```python
from build123d import *

# Parameters (mm, degrees)
F1_DEPTH = 609.6


with BuildPart() as f1:
    # F0 (on Right) → F1 (new body)
    with BuildSketch(Plane.YZ):
        with BuildLine():
            Line((-59.69, 12.737884), (-53.34, 12.737884))
            ThreePointArc((-53.34, 12.737884), (-56.515, 14.642884), (-59.69, 12.737884))
        make_face()
        with BuildLine():
            ThreePointArc((-118.11, 12.737884), (-121.285, 14.642884), (-124.46, 12.737884))
            Line((-124.46, 12.737884), (-118.11, 12.737884))
        make_face()
        with BuildLine():
            Line((-252.4125, 9.562884), (-9.525, 9.562884))
            ThreePointArc((-9.525, 9.562884), (-2.789808, 6.773076), (0, 0.037884))
            Line((0, 0.037884), (0, -11.720433))
            ThreePointArc((0, -11.720433), (-8.067335, -19.327291), (-15.187478, -10.827306))
            ThreePointArc((-15.187478, -10.827306), (-17.598242, -6.218379), (-22.768182, -6.789089))
            ThreePointArc((-22.768182, -6.789089), (-22.948389, -9.016326), (-20.72294, -9.217406))
            ThreePointArc((-20.72294, -9.217406), (-19.12196, -9.047525), (-18.340594, -10.45517))
            ThreePointArc((-18.340594, -10.45517), (-8.253725, -22.496816), (3.175, -11.720433))
            Line((3.175, -11.720433), (3.175, 0.037884))
            ThreePointArc((3.175, 0.037884), (-0.544744, 9.01814), (-9.525, 12.737884))
            Line((-9.525, 12.737884), (-20.32, 12.737884))
            Line((-20.32, 12.737884), (-21.082, 12.737884))
            Line((-21.082, 12.737884), (-21.844, 12.737884))
            Line((-21.844, 12.737884), (-22.606, 12.737884))
            Line((-22.606, 12.737884), (-23.368, 12.737884))
            Line((-23.368, 12.737884), (-24.13, 12.737884))
            Line((-24.13, 12.737884), (-24.892, 12.737884))
            Line((-24.892, 12.737884), (-25.654, 12.737884))
            Line((-25.654, 12.737884), (-26.416, 12.737884))
            Line((-26.416, 12.737884), (-27.178, 12.737884))
            Line((-27.178, 12.737884), (-27.94, 12.737884))
            Line((-27.94, 12.737884), (-53.34, 12.737884))
            Line((-53.34, 12.737884), (-59.69, 12.737884))
            Line((-59.69, 12.737884), (-85.09, 12.737884))
            Line((-85.09, 12.737884), (-85.852, 12.737884))
            Line((-85.852, 12.737884), (-86.614, 12.737884))
            Line((-86.614, 12.737884), (-87.376, 12.737884))
            Line((-87.376, 12.737884), (-88.138, 12.737884))
            Line((-88.138, 12.737884), (-88.9, 12.737884))
            Line((-88.9, 12.737884), (-89.662, 12.737884))
            Line((-89.662, 12.737884), (-90.424, 12.737884))
            Line((-90.424, 12.737884), (-91.186, 12.737884))
            Line((-91.186, 12.737884), (-91.948, 12.737884))
            Line((-91.948, 12.737884), (-92.71, 12.737884))
            Line((-92.71, 12.737884), (-118.11, 12.737884))
            Line((-118.11, 12.737884), (-124.46, 12.737884))
            Line((-124.46, 12.737884), (-149.86, 12.737884))
            Line((-149.86, 12.737884), (-150.622, 12.737884))
            Line((-150.622, 12.737884), (-151.384, 12.737884))
            Line((-151.384, 12.737884), (-152.146, 12.737884))
            Line((-152.146, 12.737884), (-152.908, 12.737884))
            Line((-152.908, 12.737884), (-153.67, 12.737884))
            Line((-153.67, 12.737884), (-154.432, 12.737884))
            Line((-154.432, 12.737884), (-155.194, 12.737884))
            Line((-155.194, 12.737884), (-155.956, 12.737884))
            Line((-155.956, 12.737884), (-156.718, 12.737884))
            Line((-156.718, 12.737884), (-157.48, 12.737884))
            Line((-157.48, 12.737884), (-182.88, 12.737884))
            Line((-182.88, 12.737884), (-189.23, 12.737884))
            Line((-189.23, 12.737884), (-214.63, 12.737884))
            Line((-214.63, 12.737884), (-215.392, 12.737884))
            Line((-215.392, 12.737884), (-216.154, 12.737884))
            Line((-216.154, 12.737884), (-216.916, 12.737884))
            Line((-216.916, 12.737884), (-217.678, 12.737884))
            Line((-217.678, 12.737884), (-218.44, 12.737884))
            Line((-218.44, 12.737884), (-219.202, 12.737884))
            Line((-219.202, 12.737884), (-219.964, 12.737884))
            Line((-219.964, 12.737884), (-220.726, 12.737884))
            Line((-220.726, 12.737884), (-221.488, 12.737884))
            Line((-221.488, 12.737884), (-222.25, 12.737884))
            Line((-222.25, 12.737884), (-247.65, 12.737884))
            Line((-247.65, 12.737884), (-254, 12.737884))
            Line((-254, 12.737884), (-254, 11.150384))
            ThreePointArc((-254, 11.150384), (-253.535032, 10.027852), (-252.4125, 9.562884))
        make_face()
        with BuildLine():
            ThreePointArc((-247.65, 12.737884), (-250.825, 14.642884), (-254, 12.737884))
            Line((-254, 12.737884), (-247.65, 12.737884))
        make_face()
        with BuildLine():
            ThreePointArc((-182.88, 12.737884), (-186.055, 14.642884), (-189.23, 12.737884))
            Line((-189.23, 12.737884), (-182.88, 12.737884))
        make_face()
        Polygon((-85.852, 12.737884), (-85.09, 12.737884), (-85.852, 13.753884), align=None)
        Polygon((-21.082, 12.737884), (-20.32, 12.737884), (-21.082, 13.753884), align=None)
        Polygon((-222.25, 13.753884), (-222.25, 12.737884), (-221.488, 12.737884), align=None)
        Polygon((-21.844, 12.737884), (-21.082, 12.737884), (-21.844, 13.753884), align=None)
        Polygon((-150.622, 13.753884), (-150.622, 12.737884), (-149.86, 12.737884), align=None)
        Polygon((-151.384, 13.753884), (-151.384, 12.737884), (-150.622, 12.737884), align=None)
        Polygon((-221.488, 13.753884), (-221.488, 12.737884), (-220.726, 12.737884), align=None)
        Polygon((-86.614, 12.737884), (-85.852, 12.737884), (-86.614, 13.753884), align=None)
        Polygon((-26.416, 12.737884), (-25.654, 12.737884), (-26.416, 13.753884), align=None)
        Polygon((-27.178, 12.737884), (-26.416, 12.737884), (-27.178, 13.753884), align=None)
        Polygon((-152.908, 13.753884), (-152.908, 12.737884), (-152.146, 12.737884), align=None)
        Polygon((-157.48, 13.753884), (-157.48, 12.737884), (-156.718, 12.737884), align=None)
        Polygon((-215.392, 13.753884), (-215.392, 12.737884), (-214.63, 12.737884), align=None)
        Polygon((-92.71, 13.753884), (-92.71, 12.737884), (-91.948, 12.737884), align=None)
        Polygon((-89.662, 12.737884), (-88.9, 12.737884), (-89.662, 13.753884), align=None)
        Polygon((-155.194, 13.753884), (-155.194, 12.737884), (-154.432, 12.737884), align=None)
        Polygon((-153.67, 13.753884), (-153.67, 12.737884), (-152.908, 12.737884), align=None)
        Polygon((-91.948, 12.737884), (-91.186, 12.737884), (-91.948, 13.753884), align=None)
        Polygon((-87.376, 12.737884), (-86.614, 12.737884), (-87.376, 13.753884), align=None)
        Polygon((-24.13, 12.737884), (-23.368, 12.737884), (-24.13, 13.753884), align=None)
        Polygon((-27.94, 12.737884), (-27.178, 12.737884), (-27.94, 13.753884), align=None)
        Polygon((-90.424, 12.737884), (-89.662, 12.737884), (-90.424, 13.753884), align=None)
        Polygon((-23.368, 12.737884), (-22.606, 12.737884), (-23.368, 13.753884), align=None)
        Polygon((-218.44, 13.753884), (-218.44, 12.737884), (-217.678, 12.737884), align=None)
        Polygon((-219.202, 13.753884), (-219.202, 12.737884), (-218.44, 12.737884), align=None)
        Polygon((-216.154, 13.753884), (-216.154, 12.737884), (-215.392, 12.737884), align=None)
        Polygon((-155.956, 13.753884), (-155.956, 12.737884), (-155.194, 12.737884), align=None)
        Polygon((-219.964, 13.753884), (-219.964, 12.737884), (-219.202, 12.737884), align=None)
        Polygon((-88.138, 12.737884), (-87.376, 12.737884), (-88.138, 13.753884), align=None)
        Polygon((-88.9, 12.737884), (-88.138, 12.737884), (-88.9, 13.753884), align=None)
        Polygon((-24.892, 12.737884), (-24.13, 12.737884), (-24.892, 13.753884), align=None)
        Polygon((-152.146, 13.753884), (-152.146, 12.737884), (-151.384, 12.737884), align=None)
        Polygon((-220.726, 13.753884), (-220.726, 12.737884), (-219.964, 12.737884), align=None)
        Polygon((-216.916, 13.753884), (-216.916, 12.737884), (-216.154, 12.737884), align=None)
        Polygon((-156.718, 13.753884), (-156.718, 12.737884), (-155.956, 12.737884), align=None)
        Polygon((-154.432, 13.753884), (-154.432, 12.737884), (-153.67, 12.737884), align=None)
        Polygon((-217.678, 13.753884), (-217.678, 12.737884), (-216.916, 12.737884), align=None)
        Polygon((-25.654, 12.737884), (-24.892, 12.737884), (-25.654, 13.753884), align=None)
        Polygon((-22.606, 12.737884), (-21.844, 12.737884), (-22.606, 13.753884), align=None)
        Polygon((-91.186, 12.737884), (-90.424, 12.737884), (-91.186, 13.753884), align=None)
    extrude(amount=F1_DEPTH)


solid = f1.part
```
Geometry check sheet. Reference: the model listing, model coordinates, mm. A direction names the side the tool comes from. Coordinates: 2 decimals unless noted, no trailing zeros. Write each loop counter-clockwise with the first axis right and the second up, starting at its lowest first coordinate (ties: lowest second). Pieces come first, ordered by that corner, then holes. Notation, with made-up numbers: M -27,82 L -19,82 A15 cw -19,90 Z; hole C 32,74.25 d7. An arc over 180 degrees is marked long. One line per item, written item: value. Start each with the question number.
(1) Tool access check on faces 1 (the face through (301, -40, 12.738)), 2 (the face through (609.6, -116, 10)), 3 (the face through (300.533, -7.894, -19.336)). Record the directions out of +Z, -Z, +X, -X, +Y, -Y that give a thin tool (end or side, any length) a straight path to the whole face; none if there is none.
(2) Sectioned sample at A-A, the plane y = -200. Enter the section's corners in (x, z), and give its area (3 significant figures).
(3) Depth check by flat-ended pin: pin 1 (1.5 mm diameter, centred on x = 545.5, y = -27, fed in from -Z); pin 2 (2 mm diameter, centred on x = 332.5, z = 5.5, fed in from +Y); pin 3 (5 mm diameter, centred on x = 407.5, z = 9, fed in from +Y). Enter the tip coordinate at first touch or a pass-through.
(4) Release check for a two-part mould opening along Y. For faces 4 (the face through (301, -137, 12.738)), 5 (the face through (300.53, -8.5, -22.48)), 6 (the face through (301, -15, 12.738)) record: released by +Y, released by -Y, zero draft, split by the parting line, or undercut.
(5) Scan lines: line 1 along Y through (x, z) = (347.5, -13); line 2 along Y through (x, z) = (380.5, -2.5) (3 decimals); line 3 along Z through (x, y) = (548, -110). Record each from-to range of solid material in increasing order. Write a range as [from, to].
Filled sheet:
1. face 1: +Z, +X, -X
1. face 2: +Z, -Z, +X, +Y, -Y
1. face 3: +X, -X
2. outline: M 0,9.56 L 609.6,9.56 L 609.6,12.74 L 0,12.74 Z
2. area: 1,940 mm²
3. pin 1: z = 9.56
3. pin 2: y = 2.37
3. pin 3: y = 1.41
4. face 4: undercut
4. face 5: split by the parting line
4. face 6: zero draft
5. line 1: [-18.34, -15.13], [-0.11, 3.1]
5. line 2: [0, 3.175]
5. line 3: [9.56, 12.74]
